Model file for the job. Use its own axes, mm. A direction names the side the tool comes from. Round coordinates to 2 decimals unless told otherwise and drop trailing zeros. Order: outer loops, then holes, each group sorted by start corner. A loop starts at its lowest first (then second) coordinate and runs counter-clockwise, first axis right, second up. Notation, with made-up numbers: M -14,20.25 L 12,20.25 A24 cw 12,46.25 Z; hole C 40,86.5 d8. An arc over 180 degrees is marked long. Return JSON: item names as keys, results as strings. Group by question number.
Item 1: Slice it at D-D on x = 7.45. Write the cut outline in (y, z), then the cut area to 3 significant figures.
Item 2: Pin check, flat tips, straight feed: pin 1 Ø8 at (y, z) = (9, 13.5) entering from -X; pin 2 Ø3 at (y, z) = (9.5, 18.5) entering from +X; pin 3 Ø6.5 at (x, z) = (16, -15.5) entering from +Y; pin 4 Ø6 at (y, z) = (7, -8) entering from -X. Stop position of each tip, or through.
Item 3: Slice it at C-C on y = 6.25. Give the number of separate pieces and of enclosed holes in the cut face, then the cut area to 3 significant figures.
Item 4: Which spindle directions (+Z, -Z, +X, -X, +Y, -Y) get a long thin tool onto all of the face, cutting with end or side? Do faces 1 (the face through (21.7, 7, -16)), 2 (the face through (0, 10, 0)), 3 (the face through (0, 5, 2)). Say none if no direction does.
Item 5: Pull direction X, two halves, no side cores. Call faces 4 (the face through (20.9, 7, 16)), 5 (the face through (16, 13, -16)), 6 (the face through (0, 7, 21.05)): pulls with the +X half, pulls with the -X half, needs draft (parallel to the pull), parting line crosses it, or undercut.
Item 6: Slice it at A-A on z = -11.05. Write the cut outline in (x, y).
Item 7: Slice it at B-B on x = -18.5. Write the cut outline in (y, z), then the cut area to 3 significant figures.
Item 8: Probe line 1 along Z through (x, y) = (11.7, 0.75); line 2 along X through (y, z) = (0.65, -11.05); line 3 along Z through (x, y) = (1, 3). List the from-to ranges inside material, lowest first.
from build123d import *

# Parameters (mm, degrees)
SKETCH1_W           = 43.8
SKETCH1_H           = 42.5
BOSS_EXTRUDE1_DEPTH = 1
SKETCH2_W           = 41.8
SKETCH2_H           = 10.3
BOSS_EXTRUDE2_DEPTH = 12.4
SKETCH3_R           = 4.15
BOSS_EXTRUDE3_DEPTH = 12.4
SKETCH4_W           = 11
SKETCH4_H           = 6
BOSS_EXTRUDE4_DEPTH = 12
SKETCH5_W           = 6
SKETCH5_H           = 6
BOSS_EXTRUDE5_DEPTH = 4
SKETCH6_R           = 1.5
BOSS_EXTRUDE6_DEPTH = 5
SKETCH7_R           = 1.55
CUT_EXTRUDE1_DEPTH  = 2
FILLET1_R           = 0.6


with BuildPart() as part:
    # Sketch1 → Boss-Extrude1 (new body)
    with BuildSketch(Plane(origin=(0, 0, 0), x_dir=(1, 0, 0), z_dir=(0, 1, 0))):
        Rectangle(SKETCH1_W, SKETCH1_H)
    extrude(amount=BOSS_EXTRUDE1_DEPTH)

    # Sketch2 → Boss-Extrude2 (add)
    with BuildSketch(Plane(origin=(0, 1, 0), x_dir=(1, 0, 0), z_dir=(0, 1, 0))):
        with Locations((0, -15.9)):
            Rectangle(SKETCH2_W, SKETCH2_H)
    extrude(amount=BOSS_EXTRUDE2_DEPTH)

    # Sketch3 → Boss-Extrude3 (add)
    with BuildSketch(Plane.XY.offset(21.05)):
        with Locations((7.45, 7.55)):
            Circle(SKETCH3_R)
        with Locations((-7.45, 7.55)):
            Circle(SKETCH3_R)
    extrude(amount=BOSS_EXTRUDE3_DEPTH)

    # Sketch4 → Boss-Extrude4 (add)
    with BuildSketch(Plane(origin=(0, 1, 0), x_dir=(1, 0, 0), z_dir=(0, 1, 0))):
        with Locations((16.2, 16.25)):
            Rectangle(SKETCH4_W, SKETCH4_H)
    extrude(amount=BOSS_EXTRUDE4_DEPTH)

    # Sketch5 → Boss-Extrude5 (add)
    with BuildSketch(Plane(origin=(0, 1, 0), x_dir=(1, 0, 0), z_dir=(0, 1, 0))):
        with Locations((0, -0.25)):
            Rectangle(SKETCH5_W, SKETCH5_H)
    extrude(amount=BOSS_EXTRUDE5_DEPTH)

    # Sketch6 → Boss-Extrude6 (add)
    with BuildSketch(Plane(origin=(0, 5, 0), x_dir=(1, 0, 0), z_dir=(0, 1, 0))):
        Circle(SKETCH6_R)
    extrude(amount=BOSS_EXTRUDE6_DEPTH)

    # Sketch7 → Cut-Extrude1 (cut, through all)
    with BuildSketch(Plane(origin=(0, 1, 0), x_dir=(1, 0, 0), z_dir=(0, 1, 0))):
        with Locations((11.7, 11.05)):
            Circle(SKETCH7_R)
    extrude(amount=-CUT_EXTRUDE1_DEPTH, mode=Mode.SUBTRACT)

    # Fillet1
    fillet1_edges = [part.edges().sort_by_distance(p)[0] for p in [
        (3.3, 7.55, 33.45),
        (-11.6, 7.55, 33.45),
    ]]
    fillet(fillet1_edges, radius=FILLET1_R)


solid = part.part
Output values:
{
 "1": {"outline": "M 0,-21.25 L 1,-21.25 L 1,10.75 L 13.4,10.75 L 13.4,21.05 L 11.7,21.05 L 11.7,32.85 A0.6 ccw 11.1,33.45 L 4,33.45 A0.6 ccw 3.4,32.85 L 3.4,21.05 L 1,21.05 L 1,21.25 L 0,21.25 Z", "area": "273 mm²"},
 "2": {"pin 1": "x = -20.9", "pin 2": "x = 20.9", "pin 3": "y = 13", "pin 4": "through"},
 "3": {"separate pieces": "3", "enclosed holes": "0", "area": "699 mm²"},
 "4": {"face 1": "+Z, -Z, +X, +Y", "face 2": "-Z, +X, -X, +Y", "face 3": "+Y"},
 "5": {"face 4": "pulls with the +X half", "face 5": "needs draft", "face 6": "undercut"},
 "6": {"outline": "M -21.9,0 L 10.15,0 L 10.15,1 L -21.9,1 Z; M 13.25,0 L 21.9,0 L 21.9,1 L 13.25,1 Z"},
 "7": {"outline": "M 0,-21.25 L 1,-21.25 L 1,10.75 L 13.4,10.75 L 13.4,21.05 L 1,21.05 L 1,21.25 L 0,21.25 Z", "area": "170 mm²"},
 "8": {"line 1": "-21.25 to -12.6, -9.5 to 21.25", "line 2": "-21.9 to 10.15, 13.25 to 21.9", "line 3": "-2.75 to 3.25, 10.75 to 21.05"}
}
